Source: CAD feature listing. Evaluate the final solid. Frame: model axes, mm. A direction names the side the tool comes from. Round coordinates to 2 decimals unless told otherwise and drop trailing zeros. Return JSON: item names as keys, results as strings. Group by question number.
1) Contact query for flat-ended pins moving along their axis: P1, Ø10, axis at x = 91, z = 15, coming from the +Y side; P2, Ø5, axis at y = -17, z = -5.5, coming from the +X side; P3, Ø10, axis at x = 449, y = 21, coming from the -Z side. Output: stop coordinate, or through.
2) Ray query, line 1 (Z direction, x = 447.5, y = 32.5); line 2 (Z direction, x = 64.5, y = -6.5); line 3 (Z direction, x = 479.5, y = -30.5). Return the intervals inside material, ascending. Write a range as from..to.
3) Mould query, pull axis Y, two halves, no side actions, for faces 1 (the cylindrical face through (479.2, -35.434, -11.159)), 2 (the flat face through (451, 1, 1)), 3 (the flat face through (451, -11.9, 35.4)). Classes: pulls with the +Y half, pulls with the -Y half, needs draft (parallel to the pull), parting line crosses it, or undercut.
4) Access query for faces 4 (the cylindrical face through (480, 30.75, -19.6)), 5 (the flat face through (508.2, -27, 25)). Directions: +Z, -Z, +X, -X, +Y, -Y. A direction counts if a zero-diameter tool reaches every point of the face in a straight line with its end or side. Return the directions, or none.
```python
from build123d import *

# Parameters (mm, degrees)
SKETCH7_R           = 37.15
BOSS_EXTRUDE1_DEPTH = 57.2
SKETCH10_R          = 36.465
CUT_EXTRUDE1_DEPTH  = 57.2


with BuildPart() as part:
    # Sketch4 → Revolve1 (revolve)
    with BuildSketch(Plane.XY):
        with BuildLine():
            Line((451, 39.65), (451, 0))
            Line((451, 0), (0.000701246, 0))
            add(Edge.make_bspline(
                [(0.000701246, 0), (0.002506302, 0.004250308), (0.00680812, 0.012312245), (0.018396223, 0.026567262), (0.044870426, 0.051987464), (0.084367289, 0.083263169), (0.137290098, 0.119470755), (0.212480734, 0.165700096), (0.302732494, 0.215977448), (0.408604965, 0.270245958), (0.530135293, 0.328212169), (0.705937544, 0.407366655), (0.978806956, 0.521481954), (1.447715348, 0.70081044), (2.290942601, 0.990255514), (3.803522224, 1.450385156), (6.592175117, 2.192565449), (11.803862458, 3.39234852), (20.997899725, 5.207453532), (36.304145868, 7.801992547), (57.101225143, 10.838109762), (82.142689037, 14.064606), (109.694474906, 17.250908512), (137.276216784, 20.164082652), (164.880967367, 22.849887266), (192.504223184, 25.337299208), (220.143173378, 27.643621725), (247.795785791, 29.779575236), (275.460677162, 31.750129242), (303.136821137, 33.555775426), (330.823513329, 35.192009963), (358.520267123, 36.648600608), (382.763491855, 37.749324719), (403.549463902, 38.547560188), (420.308211797, 39.076417022), (431.587662282, 39.365684368), (440.851982053, 39.547180034), (446.650695, 39.622701869), (449.55020557, 39.646815638), (451, 39.65)],
                knots=[0, 0, 0, 0, 0, 4.0378e-05, 8.0757e-05, 0.000161513, 0.000323027, 0.00048454, 0.000646053, 0.000940145, 0.001234238, 0.001534067, 0.001833897, 0.002641117, 0.003843417, 0.005962695, 0.009698215, 0.016587688, 0.029299296, 0.053140175, 0.092371284, 0.153547186, 0.214723093, 0.275899002, 0.33707491, 0.398250818, 0.459426727, 0.520602636, 0.581778544, 0.642954453, 0.704130361, 0.765306269, 0.826482178, 0.887658087, 0.918246041, 0.948833995, 0.974416997, 0.987208499, 1, 1, 1, 1, 1], degree=4))
        make_face()
    revolve(axis=Axis((0.000701246, 0, 0), (1, 0, 0)))

    # Sketch7 → Boss-Extrude1 (add)
    with BuildSketch(Plane(origin=(451, 0, 0), x_dir=(0, 0, -1), z_dir=(1, 0, 0))):
        with Locations(Location((0, 0, 0), (0, 0, 270))):
            Circle(SKETCH7_R)
    extrude(amount=BOSS_EXTRUDE1_DEPTH)

    # Sketch10 → Cut-Extrude1 (cut)
    with BuildSketch(Plane(origin=(508.2, 0, 0), x_dir=(0, 0, -1), z_dir=(1, 0, 0))):
        Circle(SKETCH10_R)
    extrude(amount=-CUT_EXTRUDE1_DEPTH, mode=Mode.SUBTRACT)


solid = part.part
```
Geometry check:
{
 "1": {"P1": "y = 11.32", "P2": "x = 451", "P3": "z = -36.27"},
 "2": {"line 1": "-22.67..22.67", "line 2": "-9.78..9.78", "line 3": "-21.21..-19.99, 19.99..21.21"},
 "3": {"face 1": "parting line crosses it", "face 2": "undercut", "face 3": "needs draft"},
 "4": {"face 4": "+X", "face 5": "+Z, -Z, +X, +Y, -Y"}
}
